Read the model definition and answer for the solid it produces. Units are mm, in the model's axes. Give positions to 0.01 mm unless a question says otherwise; leave off trailing zeros. Write each loop counter-clockwise with the first axis right and the second up, starting at its lowest first coordinate (ties: lowest second). Pieces come first, ordered by that corner, then holes.
```python
from build123d import *

# Parameters (mm, degrees)
SKETCH1_R           = 10
BOSS_EXTRUDE1_DEPTH = 2.5
CHAMFER1_SIZE       = 2
CHAMFER1_SIZE_2     = 5.494954839


with BuildPart() as part:
    # Sketch1 → Boss-Extrude1 (new body)
    with BuildSketch(Plane.XY):
        Circle(SKETCH1_R)
    extrude(amount=BOSS_EXTRUDE1_DEPTH)

    # Sketch3 → CSK for M4 Flat Head Machine Screw1 (revolve, cut)
    with BuildSketch(Plane(origin=(0, 0, 2.5), x_dir=(0, -1, 0), z_dir=(1, 0, 0))):
        Polygon((0, 0), (0, 2.5), (2.25, 2.5), (2.25, 2.45), (4.7, 0), align=None)
    revolve(axis=Axis((0, 0, 8.85), (0, 0, -1)), mode=Mode.SUBTRACT)

    # Chamfer1
    # the kernel refuses this chamfer: 5.494954839, 2 mm, written as the material it takes off along each edge
    with BuildSketch(Plane(origin=(0, 0, 2.5), x_dir=(1, 0, 0), z_dir=(0, -1, 0))) as chamfer1_piece_1:
        Polygon((10, -CHAMFER1_SIZE), (10 - CHAMFER1_SIZE_2, 0), (10, 0), align=None)
    revolve(axis=Axis((0, 0, 2.5), (0, 0, 1)), mode=Mode.SUBTRACT)


solid = part.part
```
Item 1: Determine the mould class of faces 1 (the cylindrical face through (-2.17, -9.76, 0.25)), 2 (the conical face through (2.343, 0.52, 0.2)), 3 (the flat face through (2, -2, 0)) for opening direction Y: pulls with the +Y half, pulls with the -Y half, needs draft (parallel to the pull), parting line crosses it, or undercut.
Result set:
face 1: parting line crosses it
face 2: undercut
face 3: needs draft
Item 2: Section A-A (x = 0) is taken. Write down the section's boundary in (y, z).
Result set:
outline: (-10, 0) - (-2.25, 0) - (-2.25, 0.05) - (-4.65, 2.45) - (-10, 0.5) - close; (2.25, 0) - (10, 0) - (10, 0.5) - (4.65, 2.45) - (2.25, 0.05) - close
Item 3: Each of these flat-tipped pins is pushed along its axis until it touches: pin 1 Ø6 at (x, y) = (0, 0) entering from +Z; pin 2 Ø6 at (x, y) = (4, -3.5) entering from +Z; pin 3 Ø5 at (x, y) = (-7, 7.5) entering from +Z. Where does it stop, or does it pass through?
Result set:
pin 1: stops at z = 0.8
pin 2: stops at z = 2.45
pin 3: stops at z = 1.32
Item 4: Find the intervals of material crossed by line 1 along Y through (x, z) = (-2, 0.3); line 2 along X through (y, z) = (1, 0.25); line 3 along Y through (x, z) = (-7.5, 0.3), in increasing order.
Result set:
line 1: y = -9.8 to -1.5, 1.5 to 9.8
line 2: x = -9.95 to -2.24, 2.24 to 9.95
line 3: y = -6.61 to 6.61
Item 5: Section C-C (z = 1.05) is taken. Write down the section's boundary in (x, y).
Result set:
outline: circle Ø16.98 at (0, 0); hole circle Ø6.5 at (0, 0)
